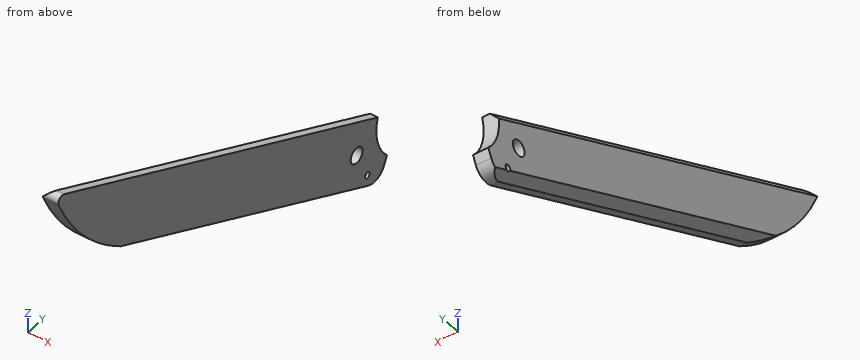
from build123d import *

# Parameters (mm, degrees)
F0_R        = 1
F0_R_2      = 2.5
F1_DEPTH    = 5
F2_T1_DEPTH = 140.5508565822
F2_T3_DEPTH = 158.1494237613


# Not quite as in the source:
# - a fillet or chamfer that OpenCascade refuses, or shapes differently, is made with other operations: its cross-section is extruded or revolved along the edge and cut away or added


with BuildPart() as f1:
    # F0 (on Right) → F1 (new body)
    with BuildSketch(Plane.YZ):
        with BuildLine():
            Line((-238.351838073, 51.1362271676), (-133.7205907933, 3.81650843))
            ThreePointArc((-133.7205907933, 3.81650843), (-129.8957188572, 3.6939702207), (-127.1044783752, 6.3119155052))
            Line((-127.1044783752, 6.3119155052), (-125.8958157643, 8.9844562534))
            ThreePointArc((-125.8958157643, 8.9844562534), (-129.9178817918, 15.9435567205), (-129.7697865993, 23.9799839275))
            Line((-129.7697865993, 23.9799839275), (-224.5101433949, 66.8265250251))
            Line((-224.5101433949, 66.8265250251), (-262.1519725075, 83.8501275596))
            ThreePointArc((-262.1519725075, 83.8501275596), (-264.0478442183, 83.5411975558), (-264.4983908426, 81.6739067294))
            ThreePointArc((-264.4983908426, 81.6739067294), (-264.4532671282, 81.571051598), (-264.4079761186, 81.4682700232))
            ThreePointArc((-264.4079761186, 81.4682700232), (-253.6243159552, 64.3742338109), (-238.351838073, 51.1362271676))
        make_face()
        with Locations((-134.1624917959, 7.5852589493)):
            Circle(F0_R, mode=Mode.SUBTRACT)
        with Locations((-138.7114049438, 17.0487332662)):
            Circle(F0_R_2, mode=Mode.SUBTRACT)
        with BuildLine():
            ThreePointArc((-264.4983908426, 81.6739067294), (-264.4565130864, 81.5696244091), (-264.4079761186, 81.4682700232))
            ThreePointArc((-264.4079761186, 81.4682700232), (-264.4532671282, 81.571051598), (-264.4983908426, 81.6739067294))
        make_face()
    extrude(amount=-F1_DEPTH)

    # F2: chamfer of 2.5 on 2 edges, made by hand

    # F2_s2 → F2_t1 (cut)
    with BuildSketch(Plane(origin=(0, -234.652694271, 106.1222128437), x_dir=(1, 0, 0), z_dir=(0, 0.9111519493, -0.4120705343))):
        Polygon((-2.5, 51.6248961977), (-5, 49.1248961977), (-5, 51.6248961977), align=None)
    extrude(amount=F2_T1_DEPTH, mode=Mode.SUBTRACT)

    # F2_s4 → F2_t3 (cut)
    with BuildSketch(Plane(origin=(0, -110.8801138075, 50.1457827883), x_dir=(1, 0, 0), z_dir=(0, -0.9111519493, 0.4120705343))):
        Polygon((-2.5, -31.6248961977), (-5, -34.1248961977), (-5, -31.6248961977), align=None)
    extrude(amount=F2_T3_DEPTH, mode=Mode.SUBTRACT)


solid = f1.part
For this review, take the finished solid that the model builds, in its own axes (mm). Round coordinates to 2 decimals unless told otherwise and drop trailing zeros. Order: outer loops, then holes, each group sorted by start corner. A loop starts at its lowest first (then second) coordinate and runs counter-clockwise, first axis right, second up. Notation, with made-up numbers: (6.5, -30) -> (44.5, -30) arc R29 ccw to (44.5, 8) -> close; hole circle Ø8 at (-5, 29). An arc over 180 degrees is marked (long way). Write item = value, one per line. Start each with the question number.
1) Take a section at D-D on y = -252.5. State the section outline as (x, z) points (3 decimals).
2) Take a section at B-B on y = -205.5. State the section outline as (x, z) points, plus the area to 3 significant figures.
3) Take a section at A-A on x = -3.7. State the section outline as (y, z) points.
4) Insertion check: pin 1 (1.6 mm diameter, centred on y = -134.16, z = 7.59, fed in from +X). The pin has a flat end and moves straight along its axis. Give the tip position at first contact, or say it passes through.
5) Take a section at C-C on z = 74.5. State the section outline as (x, y) points.
6) To check wall thickness, follow line 1 (Z direction, x = -1.85, y = -139); line 2 (Z direction, x = -3.55, y = -138.5); line 3 (Y direction, x = -2.9, z = 64). State the ranges of each line that lie inside material, in increasing order. Write a range as from..to.
Verdict:
q1.outline = (-5, 63.098) -> (0, 63.098) -> (0, 79.485) -> (-2.5, 79.485) -> (-5, 76.741) -> close
q2.outline = (-5, 39.02) -> (-2.5, 36.28) -> (0, 36.28) -> (0, 58.23) -> (-2.5, 58.23) -> (-5, 55.49) -> close
q2.area = 103 mm2
q3.outline = (-264.41, 81.47) arc R69.03 ccw to (-243.58, 54.82) -> (-130.27, 3.57) arc R5 ccw to (-127.1, 6.31) -> (-125.9, 8.98) arc R15 cw to (-130.07, 22.8) -> (-264.15, 83.44) arc R1.74 ccw to start; hole circle Ø5 at (-138.71, 17.05); hole circle Ø2 at (-134.16, 7.59)
q4.pin_1 = through
q5.outline = (-5, -260.85) -> (0, -260.85) -> (0, -241.48) -> (-2.5, -241.48) -> (-5, -247.54) -> close
q6.line_1 = 6.2..14.57, 19.53..28.15
q6.line_2 = 7.13..14.56, 19.54..26.78
q6.line_3 = -253.3..-219.23
